Here's how the part is built. I have some questions about the finished solid (model axes, mm). Face numbers are marked on the shaded views. A direction names the side the tool comes from. Coordinates: 2 decimals unless noted, no trailing zeros. Write each loop counter-clockwise with the first axis right and the second up, starting at its lowest first coordinate (ties: lowest second). Pieces come first, ordered by that corner, then holes.
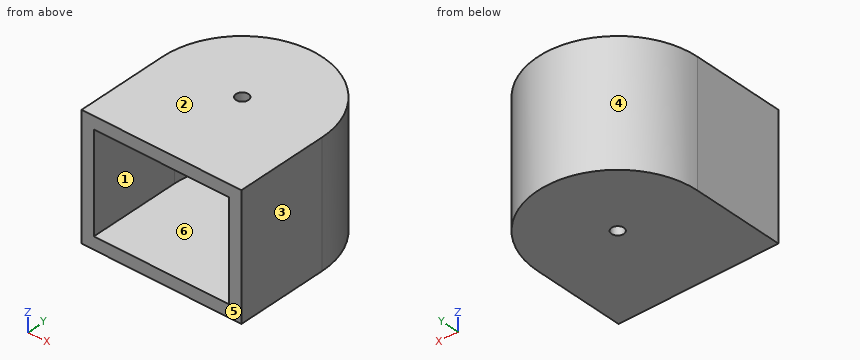
```python
from build123d import *

# Parameters (mm, degrees)
SALIENTE_EXTRUIR1_DEPTH = 100
VACIADO1_T              = -10
CROQUIS4_R              = 5
CORTAR_EXTRUIR1_DEPTH   = 130


with BuildPart() as part:
    # Croquis1 → Saliente-Extruir1 (new body)
    with BuildSketch(Plane.XY):
        with BuildLine():
            Line((-65, 0), (-65, -65))
            Line((-65, -65), (-65, -75))
            Line((-65, -75), (0, -75))
            Line((0, -75), (65, -75))
            Line((65, -75), (65, -65))
            Line((65, -65), (65, 0))
            ThreePointArc((65, 0), (0, 65), (-65, 0))
        make_face()
    extrude(amount=SALIENTE_EXTRUIR1_DEPTH)

    # Vaciado1
    vaciado1_openings = [part.faces().sort_by_distance(p)[0] for p in [
        (0, -75, 50),
    ]]
    offset(amount=VACIADO1_T, openings=vaciado1_openings, kind=Kind.INTERSECTION)

    # Croquis4 → Cortar-Extruir1 (cut)
    with BuildSketch(Plane.XY.offset(100)):
        Circle(CROQUIS4_R)
    extrude(amount=-CORTAR_EXTRUIR1_DEPTH, mode=Mode.SUBTRACT)


solid = part.part
```
1) Imagine slicing it at B-B on x = -31. Please give me the cut outline in (y, z).
Values follow:
outline: (-75, 0) - (57.13, 0) - (57.13, 100) - (-75, 100) - (-75, 90) - (45.43, 90) - (45.43, 10) - (-75, 10) - close
2) Imagine slicing it at A-A on y = -34. Please give me the cut outline in (x, z).
Values follow:
outline: (-65, 0) - (65, 0) - (65, 100) - (-65, 100) - close; hole (-55, 10) - (55, 10) - (55, 90) - (-55, 90) - close
3) Imagine slicing it at D-D on y = 29. Please give me the cut outline in (x, z).
Values follow:
outline: (-58.17, 0) - (58.17, 0) - (58.17, 100) - (-58.17, 100) - close; hole (-46.73, 10) - (46.73, 10) - (46.73, 90) - (-46.73, 90) - close
4) On a 3-axis mill with a long thin cutter (end or side, diameter ignored), from which of +Z, -Z, +X, -X, +Y, -Y can I reach the whole of each face in a straight line? I mean the marked faces 5 and 6. Say none if no direction works.
Values follow:
face 5: +Z, -Z, +X, -X, -Y
face 6: -Y
5) I need wall thicknesses on probe 1 along Y at (x, z) = (0, 5); probe 2 along X at (y, z) = (-21.5, 48); probe 3 along Z at (x, y) = (21, 27.5). Which ranges of each line are inside material? Lowest first, please.
Values follow:
probe 1: y = -75 to -5, 5 to 65
probe 2: x = -65 to -55, 55 to 65
probe 3: z = 0 to 10, 90 to 100
6) We'd pull the mould along X, two halves only. Please class the marked faces 1, 2, 3 and 4: pulls with the +X half, pulls with the -X half, needs draft (parallel to the pull), parting line crosses it, or undercut.
Values follow:
face 1: undercut
face 2: needs draft
face 3: pulls with the +X half
face 4: parting line crosses it
7) Will these pins go through, and if not, where does the flat tip stop? pin 1 (4 mm diameter, centred on x = -2, z = 84, fed in from -Y); pin 2 (8 mm diameter, centred on x = -43.5, z = 44, fed in from +Y); pin 3 (4 mm diameter, centred on x = -36.5, z = 18.5, fed in from +Y).
Values follow:
pin 1: stops at y = 54.85
pin 2: stops at y = 51.62
pin 3: stops at y = 55.09
8) Imagine slicing it at C-C on z = 57. Please give me the cut outline in (x, y).
Values follow:
outline: (-65, -75) - (-55, -75) - (-55, 0) arc R55 cw to (55, 0) - (55, -75) - (65, -75) - (65, 0) arc R65 ccw to (-65, 0) - close
